```python
from build123d import *

# Parameters (mm, degrees)
F1_DEPTH = 20
F3_DEPTH = 43.4
F5_DEPTH = 5
F6_R     = 5
F8_SIZE  = 5


# Not quite as in the source:
# - a feature names something its author has since deleted; it is built from what else it names


with BuildPart() as f1:
    # F0 (on Front) → F1 (new body, symmetric)
    with BuildSketch(Plane.XZ):
        Polygon((20, 10), (-20, 10), (-26.2878760695, 4.5041712001), (-52.2599183023, 4.5041712001), (-52.2599183023, -4.38100053), (-26.2878760695, -4.38100053), (-20, -10), (20, -10), (40.3509177268, -10), (51.457375288, -4.1727770417), (75.5315572023, -4.1727770417), (75.5315572023, 2.809499735), (51.457375288, 2.809499735), (40.3509177268, 13.9019489288), (25.6562046707, 13.9019489288), align=None)
    extrude(amount=F1_DEPTH, both=True)

    # F2 (on face) → F3 (cut, symmetric)
    with BuildSketch(Plane.XY.offset(10)):
        Polygon((-20, 18.0594865233), (20, 18.0594865233), (25.6562046707, 20), (40.3509177268, 20), (51.457375288, 9.7775636241), (82.4265927076, 9.7775636241), (82.4265927076, -9.7775636241), (51.457375288, -9.7775636241), (40.3509177268, -20), (25.6562046707, -20), (20, -18.0594865233), (-20, -18.0594865233), (-26.2878760695, -9.8739182577), (-73.8637112081, -9.8739182577), (-73.8637112081, -40.0371998549), (108.4082424641, -42.2960631549), (105.6976020336, 36.3123118877), (-67.5570517778, 60.9338954091), (-73.8637112081, 9.8739182577), (-26.2878760695, 9.8739182577), align=None)
    extrude(amount=F3_DEPTH, both=True, mode=Mode.SUBTRACT)

    # F4 (on Top) → F5 (join, symmetric)
    with BuildSketch(Plane.XY):
        Polygon((17.8880691528, -22.8056833148), (17.8880691528, -14.7547144443), (11.4664630964, -14.3713355064), (7.1534435265, -30.7608079165), align=None)
        Polygon((-5.6897685863, -14.7547144443), (-11.1529268324, -14.7547144443), (-23.9961370826, -24.4350470603), (-23.0376925319, -32.9652391374), (-8.6609609425, -24.4350470603), align=None)
        Polygon((-8.6609609425, 24.4350470603), (-23.0376925319, 32.9652391374), (-23.9961370826, 24.4350470603), (-11.1529268324, 14.7547144443), (-5.6897685863, 14.7547144443), align=None)
        Polygon((7.1534435265, 30.7608079165), (11.4664630964, 14.3713355064), (17.8880691528, 14.7547144443), (17.8880691528, 22.8056833148), align=None)
    extrude(amount=F5_DEPTH, both=True)

    # F6
    f6_edges = [f1.edges().sort_by_distance(p)[0] for p in [
        (-52.259918, 9.873918, 0.061585),
        (75.531557, 9.777564, -0.681639),
        (75.531557, -9.777564, -0.681639),
        (-52.259918, -9.873918, 0.061585),
    ]]
    fillet(f6_edges, radius=F6_R)

    # F8
    f8_edges = [f1.edges().sort_by_distance(p)[0] for p in [
        (33.003561, -20, 13.901949),
        (33.003561, 20, 13.901949),
    ]]
    chamfer(f8_edges, length=F8_SIZE)


solid = f1.part
```
Geometry: final body of the model. Coordinates: model frame, mm. A direction names the side the tool comes from. Round coordinates to 2 decimals unless told otherwise and drop trailing zeros. Loops run counter-clockwise (first coordinate to the right, second up) from the corner with the lowest first, then second, coordinate; pieces in that order, holes last. Notation, with made-up numbers: (-11, -14.5) -> (33, -14.5) arc R15 ccw to (33, 2.5) -> close; hole circle Ø8 at (-23, 57.25). An arc over 180 degrees is marked (long way). Write each question's results on one line, items separated by ' | '.
Item 1: Cut plane A-A on y = 26.5. Return the cut outline in (x, z).
Answers below:
outline: (-23.76, -5) -> (-12.14, -5) -> (-12.14, 5) -> (-23.76, 5) -> close; (8.27, -5) -> (12.9, -5) -> (12.9, 5) -> (8.27, 5) -> close
Item 2: Cut plane B-B on x = 35. Return the cut outline in (y, z), and give its area (3 significant figures).
Answers below:
outline: (-20, -10) -> (20, -10) -> (20, 8.9) -> (15, 13.9) -> (-15, 13.9) -> (-20, 8.9) -> close | area: 931 mm²
Item 3: Cut plane C-C on y = -2. Return the cut outline in (x, z).
Answers below:
outline: (-52.26, -4.38) -> (-26.29, -4.38) -> (-20, -10) -> (40.35, -10) -> (51.46, -4.17) -> (75.53, -4.17) -> (75.53, 2.81) -> (51.46, 2.81) -> (40.35, 13.9) -> (25.66, 13.9) -> (20, 10) -> (-20, 10) -> (-26.29, 4.5) -> (-52.26, 4.5) -> close
Item 4: Cut plane D-D on y = -27.5. Return the cut outline in (x, z).
Answers below:
outline: (-23.65, -5) -> (-13.83, -5) -> (-13.83, 5) -> (-23.65, 5) -> close; (8.01, -5) -> (11.55, -5) -> (11.55, 5) -> (8.01, 5) -> close
Item 5: Line query: probe 1 along Y at (x, z) = (-30.5, 1.25); probe 2 along Y at (x, z) = (51.5, -1.25); probe 3 along X at (y, z) = (28, 1). Output: solid intervals per line, ascending. Write a range as [from, to].
Answers below:
probe 1: y = [-9.87, 9.87] | probe 2: y = [-9.78, 9.78] | probe 3: x = [-23.6, -14.67], [7.88, 10.88]
Item 6: Set-up query: faces 4 (the face through (-37, -9.874, 0)), 5 (the face through (17.888, -20, 0)), 6 (the face through (-22.401, -14.934, 0.14)), 7 (the face through (33, -20, 0)), 8 (the face through (63, 0, -4.173)). Return all of +Z, -Z, +X, -X, +Y, -Y with unobstructed straight access to the full face (end or side cutting, diameter ignored); none if empty.
Answers below:
face 4: +Z, -Z, -X, -Y | face 5: +Z, -Z, -Y | face 6: +Z, -Z, -X | face 7: +Z, -Z, +X, -Y | face 8: -Z, +X, +Y, -Y
Item 7: Pin query (flat end, axial travel): pin 1 Ø12 at (x, y) = (45.5, 6.5) entering from +Z; pin 2 Ø1 at (x, z) = (3, 9.5) entering from +Y; pin 3 Ø5.5 at (x, y) = (10.5, 24) entering from -Z; pin 4 Ø5 at (y, z) = (-21.5, 0.5) entering from +X. Return the tip coordinate at first contact, or that it passes through.
Answers below:
pin 1: stops at z = 13.9 | pin 2: stops at y = 18.06 | pin 3: stops at z = -5 | pin 4: stops at x = 41.44
Item 8: Pull-direction query (Y, two-part tool) for faces 1 (the face through (-19.708, -21.203, -0.07)), 2 (the face through (44.75, -15.95, 0.8)), 3 (the face through (45.98, -0.25, 8.28)); classes: pulls with the +Y half, pulls with the -Y half, needs draft (parallel to the pull), parting line crosses it, or undercut.
Answers below:
face 1: undercut | face 2: pulls with the -Y half | face 3: needs draft
